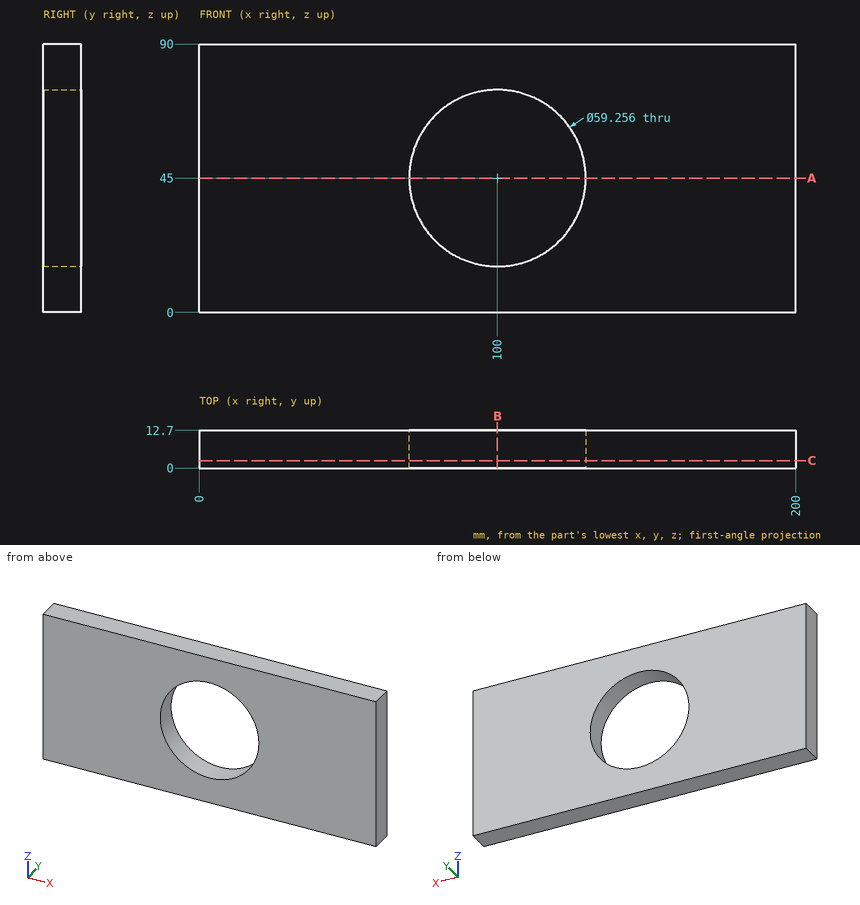
The figure shows three views and two pictorial views of one solid part (mm, origin at its lowest corner). Answer the questions. Coordinates: 2 decimals unless noted, no trailing zeros. Write each loop counter-clockwise with the first axis right and the second up, starting at its lowest first coordinate (ties: lowest second). Pieces come first, ordered by that corner, then holes.
1. Consider line 1 along X through (y, z) = (4.5, 44.5); line 2 along Z through (x, y) = (100, 4.75); line 3 along X through (y, z) = (0.5, 19) (1 decimal). Determine where each line is inside the solid, lowest interval first.
Results list:
line 1: x = 0 to 70.38, 129.62 to 200
line 2: z = 0 to 15.37, 74.63 to 90
line 3: x = 0 to 85.8, 114.2 to 200
2. The part is cut by section C-C, the plane y = 2.5. Write down the section's boundary in (x, z), and give its area (3 significant figures).
Results list:
outline: (0, 0) - (200, 0) - (200, 90) - (0, 90) - close; hole circle Ø59.26 at (100, 45)
area: 15,200 mm2
3. The part is cut by section A-A, the plane z = 45. Write down the section's boundary in (x, y), and give its area (3 significant figures).
Results list:
outline: (0, 0) - (70.37, 0) - (70.37, 12.7) - (0, 12.7) - close; (129.63, 0) - (200, 0) - (200, 12.7) - (129.63, 12.7) - close
area: 1,790 mm2
4. The part is cut by section B-B, the plane x = 100. Write down the section's boundary in (y, z).
Results list:
outline: (0, 0) - (12.7, 0) - (12.7, 15.37) - (0, 15.37) - close; (0, 74.63) - (12.7, 74.63) - (12.7, 90) - (0, 90) - close
